Can you work these out from the model? Positions are in its coordinate system, mm. Face numbers are marked on the shaded views. A direction names the side the tool comes from. Give positions to 0.01 mm unless a question says otherwise; leave off trailing zeros. Order: outer loops, then holes, each group sorted by start corner. A loop starts at its lowest first (then second) coordinate and runs counter-clockwise, first axis right, second up. Notation, with made-up numbers: (3, 45) -> (18, 45) arc R12 cw to (18, 53) -> close; hole circle Ø10 at (-23, -6.5). An arc over 180 degrees is marked (long way). Answer as CSV lines item,"result".
```python
from build123d import *

# Parameters (mm, degrees)
SKETCH_3_W          = 12.8
SKETCH_3_H          = 6
CUT_EXTRUDE_1_DEPTH = 82.240384046
SKETCH_4_R          = 6
CUT_EXTRUDE_2_DEPTH = 82.240384046
SKETCH_5_R          = 10
CUT_EXTRUDE_3_DEPTH = 101


with BuildPart() as part:
    # 草图1 → 旋转1 (revolve)
    with BuildSketch(Plane(origin=(0, 0, 0), x_dir=(1, 0, 0), z_dir=(0, 1, 0)), mode=Mode.PRIVATE) as revolve_1_sk:
        Polygon((0, 20), (20, 20), (20, 5), (40, 5), (40, 15), (50, 15), (50, -15), (40, -15), (40, -5), (20, -5), (20, -20), (0, -20), align=None)
    revolve(revolve_1_sk.sketch.rotate(Axis((0, 0, -20), (0, 0, 1)), 180), axis=Axis((0, 0, -20), (0, 0, 1)))

    # 草图2 → 切除-旋转1 (revolve, cut)
    with BuildSketch(Plane(origin=(0, 0, 0), x_dir=(1, 0, 0), z_dir=(0, 1, 0)), mode=Mode.PRIVATE) as cut_revolve_1_sk:
        Polygon((42, -3.75465), (51, -0.65567), (51, -13.34433), (42, -10.24535), align=None)
        Polygon((42, 3.75465), (51, 6.55567), (51, 13.34433), (42, 10.24535), align=None)
    revolve(cut_revolve_1_sk.sketch.rotate(Axis((0, 0, -20), (0, 0, 1)), 180), axis=Axis((0, 0, -20), (0, 0, 1)), mode=Mode.SUBTRACT)

    # 草图3 → 切除-拉伸1 (cut, through all)
    with BuildSketch(Plane.XY.offset(20)):
        with Locations((6.4, 0)):
            Rectangle(SKETCH_3_W, SKETCH_3_H)
    extrude(amount=-CUT_EXTRUDE_1_DEPTH, mode=Mode.SUBTRACT)

    # 草图4 → 切除-拉伸2 (cut, through all)
    with BuildSketch(Plane.XY.offset(20)):
        with Locations((30, 0)):
            Circle(SKETCH_4_R)
        with Locations((0, 30)):
            Circle(SKETCH_4_R)
        with Locations((-30, 0)):
            Circle(SKETCH_4_R)
        with Locations((0, -30)):
            Circle(SKETCH_4_R)
    extrude(amount=-CUT_EXTRUDE_2_DEPTH, mode=Mode.SUBTRACT)

    # 草图5 → 切除-拉伸3 (cut, symmetric)
    with BuildSketch(Plane.XY.offset(20)):
        Circle(SKETCH_5_R)
    extrude(amount=CUT_EXTRUDE_3_DEPTH, both=True, mode=Mode.SUBTRACT)


solid = part.part
```
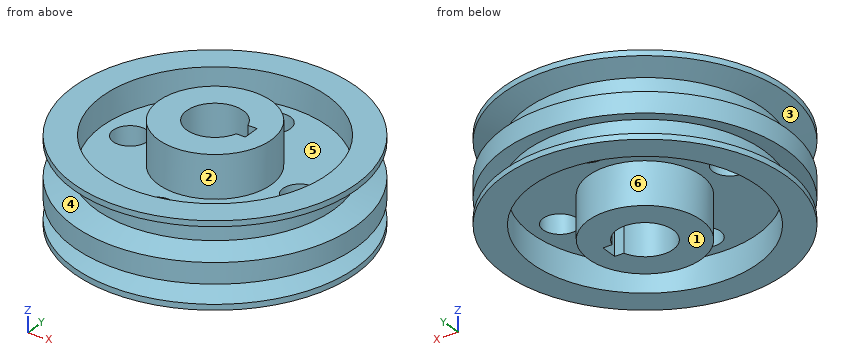
Item 1: We'd pull the mould along Z, two halves only. Please class the marked faces 1, 2 and 3: released by +Z, released by -Z, zero draft, split by the parting line, or undercut.
Numbers:
face 1,"released by -Z"
face 2,"zero draft"
face 3,"undercut"
Item 2: Please list where these lines run through material, in increasing order: line 1 along Y through (x, z) = (0, 9); line 2 along X through (y, z) = (-4, 7); line 3 along Z through (x, y) = (8, 33.5).
Numbers:
line 1,"y = -42 to -40, -20 to -10, 10 to 20, 40 to 42"
line 2,"x = -41.81 to -39.8, -19.6 to -9.17, 9.17 to 19.6, 39.8 to 41.81"
line 3,"z = -5 to 5"
Item 3: Imagine slicing it at B-B, the plane x = 0. Give the number of separate pieces and of enclosed holes in the cut face, then the cut area to 3 significant figures.
Numbers:
separate pieces,"4"
enclosed holes,"0"
area,"1,310 mm²"
Item 4: For pin 1 (15.5 mm diameter, centred on x = -30, y = 0, fed in from -Z); pin 2 (1.5 mm diameter, centred on x = 21.5, z = -2.5, fed in from -Y); pin 3 (1 mm diameter, centred on x = -22, z = 7, fed in from -Y); pin 4 (10 mm diameter, centred on x = 0, y = -1.5, fed in from +Z), each with a flat end and sliding along its axis, tell me the tip position at first contact or that it passes through.
Numbers:
pin 1,"stops at z = -5"
pin 2,"stops at y = -45.49"
pin 3,"stops at y = -36.08"
pin 4,"passes through"
Item 5: For the marked faces 4, 5 and 6, which set-ups out of +Z, -Z, +X, -X, +Y, -Y let a thin tool reach every point of the face, with its end or its side?
Numbers:
face 4,"none"
face 5,"+Z"
face 6,"-Z"
Item 6: Imagine slicing it at A-A, the plane z = -1. Please give me the cut outline in (x, y), then the cut area to 3 significant figures.
Numbers:
outline,"circle Ø100 at (0, 0); hole circle Ø12 at (-30, 0); hole circle Ø12 at (0, -30); hole circle Ø12 at (0, 30); hole (9.54, -3) -> (12.8, -3) -> (12.8, 3) -> (9.54, 3) arc R10 ccw (long way) to start; hole circle Ø12 at (30, 0)"
area,"7,070 mm²"
